Could you check a few things on this model? Use its own coordinates, in mm. Face numbers are marked on the shaded views. Round coordinates to 2 decimals unless told otherwise and drop trailing zeros. Write each loop counter-clockwise with the first axis right and the second up, starting at its lowest first coordinate (ties: lowest second). Pieces come first, ordered by that corner, then holes. Notation, with made-up numbers: (-6, 55) -> (10, 55) arc R17 cw to (10, 74) -> close; hole circle Ø8 at (56, 59.25). An arc over 180 degrees is marked (long way). One line per question, with ' | ' between items. Start each with the question number.
1. Imagine slicing it at C-C, the plane x = 15. List the corners of the cut face in (y, z) for me.
2. Imagine slicing it at D-D, the plane z = 3.5. State how many separate pieces and enclosed holes the cut face has, and give its area (3 significant figures).
3. Imagine slicing it at B-B, the plane x = 0. List the corners of the cut face in (y, z) for me (3 decimals).
4. Imagine slicing it at A-A, the plane y = 0. List the corners of the cut face in (x, z) for me.
5. Thinking about a two-plate mould opening in X: for the marked faces 1, 2, 3 and 4, which applies, released by +X, released by -X, zero draft, split by the parting line, or undercut?
6. If I drill on line 1 along Y through (x, z) = (0, 4.45) (3 decimals); line 2 along Y through (x, z) = (1, 5); line 3 along Y through (x, z) = (-7, 2), over which ranges is the centre line in solid material (lowest first)? Write a range as [from, to].
7. For pin 1 Ø1.5 at (x, z) = (4, 4.5) entering from +Y; pin 2 Ø1 at (y, z) = (2, 2) entering from -X; pin 3 Ø5.5 at (x, y) = (0, 0) entering from +Z, each with a flat end and sliding along its axis, tell me the tip position at first contact or that it passes through.
from build123d import *

# Parameters (mm, degrees)
SKETCH_1_R          = 19.75
SKETCH_1_R_2        = 3.15
EXTRUDE_1_DEPTH     = 6
SKETCH_2_R          = 1.875
CUT_EXTRUDE_2_DEPTH = 29.567901568
FILLET_1_R          = 0.5


with BuildPart() as part:
    # Эскиз1 → Бобышка-Вытянуть1 (new body)
    with BuildSketch(Plane.XY):
        Circle(SKETCH_1_R)
        Circle(SKETCH_1_R_2, mode=Mode.SUBTRACT)
    extrude(amount=EXTRUDE_1_DEPTH)

    # Эскиз2 → Вырез-Вытянуть2 (cut, through all)
    with BuildSketch(Plane(origin=(0, 0, 0), x_dir=(-1, 0, 0), z_dir=(0, 0, -1))):
        with Locations((-14.072912811, -8.125)):
            Circle(SKETCH_2_R)
        with Locations((0, 16.25)):
            Circle(SKETCH_2_R)
        with Locations((14.072912811, -8.125)):
            Circle(SKETCH_2_R)
        with BuildLine():
            Line((-10.964367017, -17.151598034), (-9.672796655, -15.131189956))
            ThreePointArc((-9.672796655, -15.131189956), (-7.115101419, -12.493124896), (-8.435759199, -15.92198115))
            Line((-8.435759199, -15.92198115), (-9.697895423, -17.896345301))
            Line((-9.697895423, -17.896345301), (-10.964367017, -17.151598034))
        make_face()
        with BuildLine():
            Line((9.371536104, -18.07121939), (8.267596564, -15.942482607))
            ThreePointArc((8.267596564, -15.942482607), (7.261812823, -12.408421028), (9.570960555, -15.266572341))
            Line((9.570960555, -15.266572341), (10.649741954, -17.34679645))
            Line((10.649741954, -17.34679645), (9.371536104, -18.07121939))
        make_face()
        with BuildLine():
            Line((-0.919621357, -20.335903121), (-0.811292651, -17.940393219))
            ThreePointArc((-0.811292651, -17.940393219), (0.084703869, -14.376914243), (0.655408809, -18.006719754))
            Line((0.655408809, -18.006719754), (0.549548851, -20.347637377))
            Line((0.549548851, -20.347637377), (-0.919621357, -20.335903121))
        make_face()
    extrude(amount=-CUT_EXTRUDE_2_DEPTH, mode=Mode.SUBTRACT)

    # Скругление1
    fillet_1_edges = [part.edges().sort_by_distance(p)[0] for p in [
        (9.371126789, -17.385179973, 3),
        (10.637598383, -16.640432706, 3),
        (8.435759199, -15.92198115, 3),
        (9.672796655, -15.131189956, 3),
        (-10.370444112, -16.808223848, 3),
        (-9.092238262, -17.532646788, 3),
        (-9.570960555, -15.266572341, 3),
        (-8.267596564, -15.942482607, 3),
        (0.892214082, -19.729836645, 3),
        (-0.576956126, -19.741570901, 3),
        (-0.655408809, -18.006719754, 3),
        (0.811292651, -17.940393219, 3),
    ]]
    fillet(fillet_1_edges, radius=FILLET_1_R)


solid = part.part
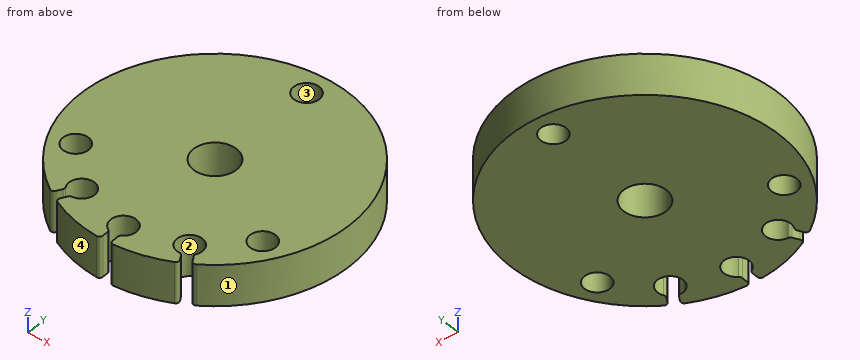
Geometry results:
1) outline: (-12.85, 0) -> (-9.75, 0) -> (-9.75, 6) -> (-12.85, 6) -> close; (-6.5, 0) -> (12.85, 0) -> (12.85, 6) -> (-6.5, 6) -> close
2) separate pieces: 1 | enclosed holes: 4 | area: 1,120 mm2
3) outline: (-14.375, 0) -> (-3.15, 0) -> (-3.15, 6) -> (-14.375, 6) -> close; (3.15, 0) -> (14.375, 0) -> (14.375, 6) -> (3.15, 6) -> close; (18.125, 0) -> (19.75, 0) -> (19.75, 6) -> (18.125, 6) -> close
4) outline: (-19.75, 0) -> (-3.15, 0) -> (-3.15, 6) -> (-19.75, 6) -> close; (3.15, 0) -> (19.75, 0) -> (19.75, 6) -> (3.15, 6) -> close
5) face 1: split by the parting line | face 2: undercut | face 3: undercut | face 4: released by -X
6) line 1: y = [-14.375, -3.15], [3.15, 14.375], [18.125, 19.75] | line 2: y = [-19.54, -17.84], [-14.66, -2.99], [2.99, 14.66], [17.84, 19.72] | line 3: y = [-18.47, -15.57], [-12.57, 18.47]
7) pin 1: stops at y = 19.48 | pin 2: stops at x = -19.69 | pin 3: passes through
